Check sheet for the drawn part. Datum: minimum x, y, z corner. Units: mm. Round coordinates to 2 decimals unless told otherwise and drop trailing zeros. Write each loop counter-clockwise with the first axis right and the second up, starting at its lowest first coordinate (ties: lowest second). Pieces come first, ordered by that corner, then holes. Notation, with made-up numbers: (55.25, -9) - (70.25, -9) arc R14 ccw to (70.25, -2) - close; hole circle Ø9 at (47.25, 12). An arc over 180 degrees is marked (long way). Answer as a JSON object with one key per item and string values. Group by question number.
Item 1: Sectioned sample at A-A on y = 127. Record the boundary of the cut face in (x, z), plus the area to 3 significant figures.
Item 2: Gauge pin test, flat ends, axial feed: P1, Ø1.2, axis at y = 62, z = 1.5, coming from the +X side; P2, Ø1.2, axis at x = 49, z = 2, coming from the -Y side; P3, Ø1.2, axis at x = 48, z = 2, coming from the +Y side. Record the tip position at first contact, or that the pin passes through.
Item 3: Thickness scan on line 1 (Y direction, x = 16, z = 0.65); line 2 (X direction, y = 16, z = 1). Record the ranges inside material, lowest first.
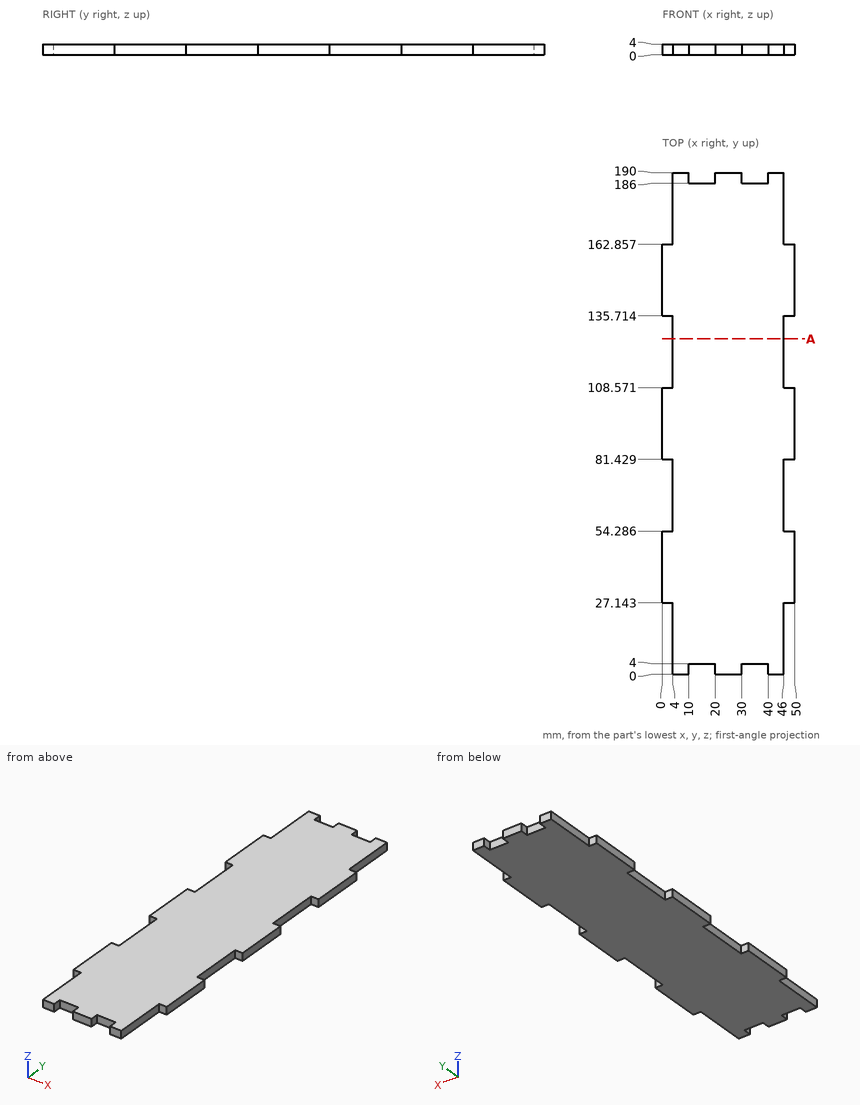
Completed:
{
 "1": {"outline": "(4, 0) - (46, 0) - (46, 4) - (4, 4) - close", "area": "168 mm²"},
 "2": {"P1": "x = 46", "P2": "y = 27.14", "P3": "y = 162.86"},
 "3": {"line 1": "4 to 186", "line 2": "4 to 46"}
}
